```python
from build123d import *

# Parameters (mm, degrees)
F1_DEPTH = 7
F2_R     = 2
F3_DEPTH = 4
F4_R     = 1.6
F5_DEPTH = 5


with BuildPart() as f1:
    # F0 (on Top) → F1 (new body)
    with BuildSketch(Plane.XY):
        with BuildLine():
            Line((32.346717088, 60.1040764009), (28.811183182, 63.6396103068))
            Line((28.811183182, 63.6396103068), (-28, 6.8284271247))
            ThreePointArc((-28, 6.8284271247), (-28.8670910053, 2.4692662705), (-25.1715728753, 0))
            Line((-25.1715728753, 0), (25.1715728753, 0))
            Line((25.1715728753, 0), (25.1715728753, 5))
            Line((25.1715728753, 5), (1.3847763109, 5))
            ThreePointArc((1.3847763109, 5), (-7.8540190143, 11.1731656763), (-5.686291501, 22.0710678119))
            Line((-5.686291501, 22.0710678119), (32.346717088, 60.1040764009))
        make_face()
    extrude(amount=F1_DEPTH)

    # F2 (on face) → F3 (cut, through all)
    with BuildSketch(Plane(origin=(-17.4142135624, 17.4142135624, 0), x_dir=(-0.7071067812, -0.7071067812, 0), z_dir=(-0.7071067812, 0.7071067812, 0))):
        with Locations((-0.372583002, 3.5)):
            Circle(F2_R)
        with Locations((-60.372583002, 3.5)):
            Circle(F2_R)
        with Locations((-30.372583002, 3.5)):
            Circle(F2_R)
    extrude(amount=-F3_DEPTH, mode=Mode.SUBTRACT)

    # F4 (on face) → F5 (cut, through all)
    with BuildSketch(Plane(origin=(0, 5, 0), x_dir=(-1, 0, 0), z_dir=(0, 1, 0))):
        with Locations((-20.1715728753, 3.5)):
            Circle(F4_R)
        with Locations((-5.1715728753, 3.5)):
            Circle(F4_R)
    extrude(amount=-F5_DEPTH, mode=Mode.SUBTRACT)


solid = f1.part
```
Part model, mm, in its own coordinate system. A direction names the side the tool comes from. Coordinates: 2 decimals unless noted, no trailing zeros. Write each loop counter-clockwise with the first axis right and the second up, starting at its lowest first coordinate (ties: lowest second). Pieces come first, ordered by that corner, then holes.
Item 1: Mould opens along Y. For faces 6 (the face through (-5, 23, 7)), 7 (the face through (30.6, 61.85, 3.45)), 8 (the face through (27.79, 59.83, 2.28)), 9 (the face through (-16.517, 15.523, 5.186)) say: released by +Y, released by -Y, zero draft, split by the parting line, or undercut.
Item 2: Slice it at D-D (y = 9.5). Write the cut outline in (x, z), and give its area (3 significant figures).
Item 3: Slice it at C-C (y = 28.5). Write the cut outline in (x, z).
Item 4: Probe line 1 (Y direction, x = 7.5, z = 4.75); line 2 (Y direction, x = 1, z = 4.25); line 3 (Y direction, x = 3, z = 2.75). List the from-to ranges inside material, lowest first.
Item 5: Which spindle directions (+Z, -Z, +X, -X, +Y, -Y) get a long thin tool onto all of the face, cutting with end or side? Do faces 1 (the face through (-28.89, 2.53, 3.45)), 2 (the face through (25.172, 2, 3)), 3 (the face through (-14.3, 14.87, 3.53)), 4 (the face through (6.35, 2.54, 4.58)), 5 (the face through (13.06, 40.82, 3.45)). Say none if no direction does.
Item 6: Slice it at A-A (z = 3.5). Write the cut outline in (x, y).
Item 7: Pin check, flat tips, straight feed: pin 1 (2.5 mm diameter, centred on x = 20.17, z = 3.5, fed in from +Y); pin 2 (2 mm diameter, centred on x = 21, z = 6, fed in from +Y); pin 3 (3.5 mm diameter, centred on x = 14.5, z = 5, fed in from +Y). Stop position of each tip, or through.
Item 8: Slice it at B-B (x = 17). Write the cut outline in (y, z).
Results found:
1. face 6: zero draft
1. face 7: released by +Y
1. face 8: undercut
1. face 9: undercut
2. outline: (-25.33, 0) - (-6.97, 0) - (-6.97, 7) - (-25.33, 7) - close
2. area: 129 mm2
3. outline: (-6.33, 0) - (0.74, 0) - (0.74, 7) - (-6.33, 7) - close
4. line 1: y = 0 to 5, 35.26 to 36.67, 37.66 to 42.33
4. line 2: y = 0 to 5.01, 28.76 to 35.83
4. line 3: y = 0 to 5, 30.76 to 37.33
5. face 1: +Z, -Z, -X
5. face 2: +Z, -Z, +X, -Y
5. face 3: none
5. face 4: -Y
5. face 5: +Z, -Z, +X
6. outline: (-28, 6.83) arc R4 ccw to (-25.17, 0) - (3.57, 0) - (3.57, 5) - (1.38, 5) arc R10 cw to (-5.69, 22.07) - (32.35, 60.1) - (28.81, 63.64) - (26.69, 61.52) - (29.52, 58.69) - (26.69, 55.86) - (23.86, 58.69) - (5.48, 40.31) - (8.31, 37.48) - (5.48, 34.65) - (2.65, 37.48) - (-15.74, 19.09) - (-12.91, 16.26) - (-15.74, 13.44) - (-18.56, 16.26) - close; (6.77, 0) - (18.57, 0) - (18.57, 5) - (6.77, 5) - close; (21.77, 0) - (25.17, 0) - (25.17, 5) - (21.77, 5) - close
7. pin 1: stops at y = 56.25
7. pin 2: stops at y = 56.83
7. pin 3: stops at y = 51.08
8. outline: (0, 0) - (5, 0) - (5, 7) - (0, 7) - close; (44.76, 0) - (51.83, 0) - (51.83, 7) - (44.76, 7) - close
